The drawing under review shows one solid part. Ordinate dimensions are in mm from its lowest x, y, z. Round coordinates to 2 decimals unless told otherwise and drop trailing zeros. Order: outer loops, then holes, each group sorted by start corner. A loop starts at its lowest first (then second) coordinate and runs counter-clockwise, first axis right, second up. Notation, with made-up numbers: (81, 41) - (121, 41) arc R8 cw to (121, 47) - close; hole circle Ø9 at (80.5, 25). An arc over 180 degrees is marked (long way). One line per question, with ' | ' between items.
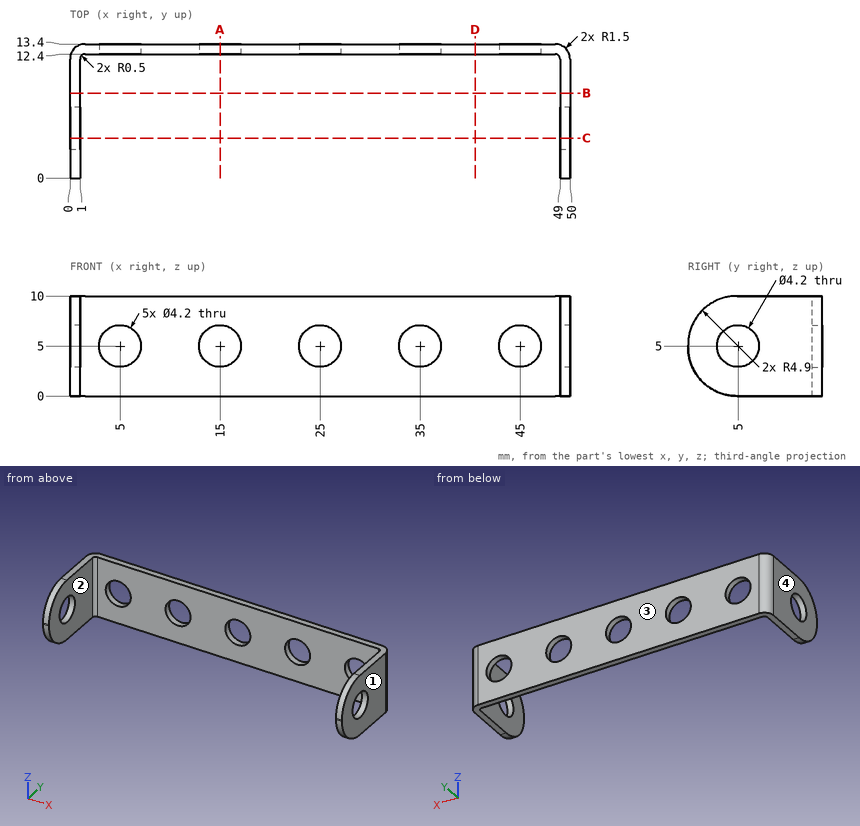
(1) We need section A-A on x = 15. State the section outline as (y, z) points.
Output values:
outline: (12.4, 0) - (13.4, 0) - (13.4, 2.9) - (12.4, 2.9) - close; (12.4, 7.1) - (13.4, 7.1) - (13.4, 10) - (12.4, 10) - close
(2) Insertion check: pin 1 (1.5 mm diameter, centred on x = 45, y = 11.5, fed in from -Z); pin 2 (5 mm diameter, centred on y = 5, z = 5, fed in from -X). Each pin has a flat end and moves straight along its axis. Give the tip position at first contact, or say it passes through.
Output values:
pin 1: through | pin 2: x = 0
(3) We need section C-C on y = 4. State the section outline as (x, z) points.
Output values:
outline: (0, 0.08) - (1, 0.08) - (1, 3.15) - (0, 3.15) - close; (0, 6.85) - (1, 6.85) - (1, 9.92) - (0, 9.92) - close; (49, 0.08) - (50, 0.08) - (50, 3.15) - (49, 3.15) - close; (49, 6.85) - (50, 6.85) - (50, 9.92) - (49, 9.92) - close
(4) For probe 1 along Z at (x, y) = (5, 12.7); probe 2 along X at (y, z) = (5, 8.75); probe 3 along Y at (x, z) = (31, 0.75), list the stretches that pass through material, from the lowest coordinate up. Write a range as [from, to].
Output values:
probe 1: [0, 2.9], [7.1, 10] | probe 2: [0, 1], [49, 50] | probe 3: [12.4, 13.4]
(5) Mouldability with a two-part tool opening along X and no side actions: class the marked faces 1, 2, 3 and 4 as released by +X, released by -X, zero draft, split by the parting line, or undercut.
Output values:
face 1: released by +X | face 2: undercut | face 3: zero draft | face 4: released by -X
(6) We need section D-D on x = 40.5. State the section outline as (y, z) points.
Output values:
outline: (12.4, 0) - (13.4, 0) - (13.4, 10) - (12.4, 10) - close
(7) We need section B-B on y = 8.5. State the section outline as (x, z) points, plus the area to 3 significant figures.
Output values:
outline: (0, 0) - (1, 0) - (1, 10) - (0, 10) - close; (49, 0) - (50, 0) - (50, 10) - (49, 10) - close | area: 20.0 mm^2
